Source: CAD feature listing. Evaluate the final solid. Frame: model axes, mm. A direction names the side the tool comes from. Give positions to 0.01 mm unless a question says otherwise; leave off trailing zeros. Order: outer loops, then holes, each group sorted by start corner. A loop starts at its lowest first (then second) coordinate and runs counter-clockwise, first axis right, second up. Notation, with made-up numbers: (16.25, 79) -> (50.25, 79) arc R15 ccw to (50.25, 96) -> close; hole circle Ø6 at (4.25, -32.5). An arc over 180 degrees is marked (long way). Answer in a Markdown table with one row per item.
```python
from build123d import *

# Parameters (mm, degrees)
SKETCH1_W                    = 255
SKETCH1_H                    = 512
BASE_FLANGE1_DEPTH           = 2.3
EDGE_FLANGE2_STRIP_W         = 13.2
EDGE_FLANGE2_STRIP_H         = 2.3
EDGE_FLANGE2_STRIP_CUT_DEPTH = 512
EDGE_FLANGE2_DEPTH           = 512
EDGE_FLANGE3_STRIP_W         = 13.2
EDGE_FLANGE3_STRIP_H         = 2.3
EDGE_FLANGE3_STRIP_CUT_DEPTH = 512
EDGE_FLANGE3_DEPTH           = 512
CUT_EXTRUDE2_START           = -10
CUT_EXTRUDE2_DEPTH           = 586.634510779
EDGE_FLANGE4_STRIP_W         = 13.2
EDGE_FLANGE4_STRIP_H         = 2.3
EDGE_FLANGE4_STRIP_CUT_DEPTH = 246.4
EDGE_FLANGE4_DEPTH           = 246.4
CUT_EXTRUDE3_REACH           = 578.501
SKETCH23_W                   = 219.6
SKETCH23_H                   = 299.3
CUT_EXTRUDE4_REACH           = 578.501
SKETCH24_W                   = 219.6
SKETCH24_H                   = 105
CUT_EXTRUDE6_REACH           = 576.175
SKETCH25_W                   = 55
SKETCH25_H                   = 40
CUT_EXTRUDE7_REACH           = 578.218
SKETCH27_W                   = 16
SKETCH27_H                   = 10
CUT_EXTRUDE8_REACH           = 578.501
SKETCH28_R                   = 5
CUT_EXTRUDE9_REACH           = 578.501
SKETCH29_R                   = 1.75
CUT_EXTRUDE10_REACH          = 578.218
SKETCH30_R                   = 3


# Sheet-metal steps are written as plain solids
with BuildPart() as part:
    # Sketch1 → Base-Flange1 (new body)
    with BuildSketch(Plane.XY):
        with Locations((127.5, 256)):
            Rectangle(SKETCH1_W, SKETCH1_H)
    extrude(amount=-BASE_FLANGE1_DEPTH)

    # Edge-Flange2 strip (across the edge) → Edge-Flange2 strip cut (cut)
    with BuildSketch(Plane(origin=(255, 0, 0), x_dir=(-1, 0, 0), z_dir=(0, 1, 0))):
        with Locations((-2.3, -1.15)):
            Rectangle(EDGE_FLANGE2_STRIP_W, EDGE_FLANGE2_STRIP_H)
    extrude(amount=EDGE_FLANGE2_STRIP_CUT_DEPTH, mode=Mode.SUBTRACT)

    # Edge-Flange2 section (across the edge) → Edge-Flange2 (add)
    with BuildSketch(Plane(origin=(255, 0, 0), x_dir=(-1, 0, 0), z_dir=(0, 1, 0))):
        with BuildLine():
            Line((0, 2), (0, 64.7))
            Line((0, 64.7), (2.3, 64.7))
            Line((2.3, 64.7), (2.3, 2))
            ThreePointArc((2.3, 2), (2.885786438, 0.585786438), (4.3, 0))
            Line((4.3, 0), (4.3, -2.3))
            ThreePointArc((4.3, -2.3), (1.259440841, -1.040559159), (0, 2))
        make_face()
    extrude(amount=EDGE_FLANGE2_DEPTH)

    # Edge-Flange3 strip (across the edge) → Edge-Flange3 strip cut (cut)
    with BuildSketch(Plane.XZ.offset(-512)):
        with Locations((-2.3, -1.15)):
            Rectangle(EDGE_FLANGE3_STRIP_W, EDGE_FLANGE3_STRIP_H)
    extrude(amount=EDGE_FLANGE3_STRIP_CUT_DEPTH, mode=Mode.SUBTRACT)

    # Edge-Flange3 section (across the edge) → Edge-Flange3 (add)
    with BuildSketch(Plane.XZ.offset(-512)):
        with BuildLine():
            Line((0, 2), (0, 64.7))
            Line((0, 64.7), (2.3, 64.7))
            Line((2.3, 64.7), (2.3, 2))
            ThreePointArc((2.3, 2), (2.885786438, 0.585786438), (4.3, 0))
            Line((4.3, 0), (4.3, -2.3))
            ThreePointArc((4.3, -2.3), (1.259440841, -1.040559159), (0, 2))
        make_face()
    extrude(amount=EDGE_FLANGE3_DEPTH)

    # Sketch17 → Cut-Extrude2 (cut)
    with BuildSketch(Plane(origin=(255, 0, 0), x_dir=(0, 0, -1), z_dir=(1, 0, 0)).offset(CUT_EXTRUDE2_START)):
        Polygon((-14.7, -1042.730361711), (-14.7, 0), (-14.7, 300), (-64.7, 512), (-64.7, 0), (-64.7, -1042.730361711), (-64.7, -3128.191085133), (-14.7, -3128.191085133), align=None)
    cut_extrude2 = extrude(amount=CUT_EXTRUDE2_DEPTH, mode=Mode.SUBTRACT)

    # Mirror6: Cut-Extrude2 across plane
    add(cut_extrude2.mirror(Plane(origin=(126.35, 0, 0), x_dir=(0, 0, 1), z_dir=(1, 0, 0))), mode=Mode.SUBTRACT)

    # Edge-Flange4 strip (across the edge) → Edge-Flange4 strip cut (cut)
    with BuildSketch(Plane(origin=(250.7, 512, 0), x_dir=(0, -1, 0), z_dir=(-1, 0, 0))):
        with Locations((-2.3, -1.15)):
            Rectangle(EDGE_FLANGE4_STRIP_W, EDGE_FLANGE4_STRIP_H)
    extrude(amount=EDGE_FLANGE4_STRIP_CUT_DEPTH, mode=Mode.SUBTRACT)

    # Edge-Flange4 section (across the edge) → Edge-Flange4 (add)
    with BuildSketch(Plane(origin=(250.7, 512, 0), x_dir=(0, -1, 0), z_dir=(-1, 0, 0))):
        with BuildLine():
            Line((0, 2), (0, 69.7))
            Line((0, 69.7), (2.3, 69.7))
            Line((2.3, 69.7), (2.3, 2))
            ThreePointArc((2.3, 2), (2.885786438, 0.585786438), (4.3, 0))
            Line((4.3, 0), (4.3, -2.3))
            ThreePointArc((4.3, -2.3), (1.259440841, -1.040559159), (0, 2))
        make_face()
    extrude(amount=EDGE_FLANGE4_DEPTH)

    # Sketch23 → Cut-Extrude3 (cut, up to next)
    with BuildSketch(Plane(origin=(0, 0, -2.3), x_dir=(-1, 0, 0), z_dir=(0, 0, -1)), mode=Mode.PRIVATE) as cut_extrude3_sk1:
        with Locations((-127.5, 209.65)):
            Rectangle(SKETCH23_W, SKETCH23_H)
    cut_extrude3_tool1 = extrude(cut_extrude3_sk1.sketch, amount=-CUT_EXTRUDE3_REACH, mode=Mode.PRIVATE) & part.part
    add(cut_extrude3_tool1.solids().sort_by_distance((127.5, 209.65, -2.3))[0], mode=Mode.SUBTRACT)

    # Sketch24 → Cut-Extrude4 (cut, up to next)
    with BuildSketch(Plane(origin=(0, 0, -2.3), x_dir=(-1, 0, 0), z_dir=(0, 0, -1)), mode=Mode.PRIVATE) as cut_extrude4_sk1:
        with Locations((-127.5, 437.8)):
            Rectangle(SKETCH24_W, SKETCH24_H)
    cut_extrude4_tool1 = extrude(cut_extrude4_sk1.sketch, amount=-CUT_EXTRUDE4_REACH, mode=Mode.PRIVATE) & part.part
    add(cut_extrude4_tool1.solids().sort_by_distance((127.5, 437.8, -2.3))[0], mode=Mode.SUBTRACT)

    # Sketch25 → Cut-Extrude6 (cut, up to next)
    with BuildSketch(Plane.XZ.offset(-509.7), mode=Mode.PRIVATE) as cut_extrude6_sk1:
        with Locations((127.5, 49.7)):
            Rectangle(SKETCH25_W, SKETCH25_H)
    cut_extrude6_tool1 = extrude(cut_extrude6_sk1.sketch, amount=-CUT_EXTRUDE6_REACH, mode=Mode.PRIVATE) & part.part
    add(cut_extrude6_tool1.solids().sort_by_distance((127.5, 509.7, 49.7))[0], mode=Mode.SUBTRACT)

    # Sketch27 → Cut-Extrude7 (cut, up to next)
    with BuildSketch(Plane(origin=(0, 512, 0), x_dir=(1, 0, 0), z_dir=(0, 1, 0)), mode=Mode.PRIVATE) as cut_extrude7_sk1:
        with Locations((108, -2.7)):
            Rectangle(SKETCH27_W, SKETCH27_H)
    cut_extrude7_tool1 = extrude(cut_extrude7_sk1.sketch, amount=-CUT_EXTRUDE7_REACH, mode=Mode.PRIVATE) & part.part
    # Sketch27 → Cut-Extrude7 (cut, up to next)
    with BuildSketch(Plane(origin=(0, 512, 0), x_dir=(1, 0, 0), z_dir=(0, 1, 0)), mode=Mode.PRIVATE) as cut_extrude7_sk2:
        with Locations((147, -2.7)):
            Rectangle(SKETCH27_W, SKETCH27_H)
    cut_extrude7_tool2 = extrude(cut_extrude7_sk2.sketch, amount=-CUT_EXTRUDE7_REACH, mode=Mode.PRIVATE) & part.part
    add(cut_extrude7_tool1.solids().sort_by_distance((108, 512, 2.7))[0], mode=Mode.SUBTRACT)
    add(cut_extrude7_tool2.solids().sort_by_distance((147, 512, 2.7))[0], mode=Mode.SUBTRACT)

    # Sketch28 → Cut-Extrude8 (cut, up to next)
    with BuildSketch(Plane(origin=(0, 0, -2.3), x_dir=(-1, 0, 0), z_dir=(0, 0, -1)), mode=Mode.PRIVATE) as cut_extrude8_sk1:
        with Locations((-127.5, 496)):
            Circle(SKETCH28_R)
    cut_extrude8_tool1 = extrude(cut_extrude8_sk1.sketch, amount=-CUT_EXTRUDE8_REACH, mode=Mode.PRIVATE) & part.part
    add(cut_extrude8_tool1.solids().sort_by_distance((127.5, 496, -2.3))[0], mode=Mode.SUBTRACT)

    # Sketch29 → Cut-Extrude9 (cut, up to next)
    with BuildSketch(Plane(origin=(0, 0, -2.3), x_dir=(-1, 0, 0), z_dir=(0, 0, -1)), mode=Mode.PRIVATE) as cut_extrude9_sk1:
        with Locations((-119.46, 496)):
            Circle(SKETCH29_R)
    cut_extrude9_tool1 = extrude(cut_extrude9_sk1.sketch, amount=-CUT_EXTRUDE9_REACH, mode=Mode.PRIVATE) & part.part
    # Sketch29 → Cut-Extrude9 (cut, up to next)
    with BuildSketch(Plane(origin=(0, 0, -2.3), x_dir=(-1, 0, 0), z_dir=(0, 0, -1)), mode=Mode.PRIVATE) as cut_extrude9_sk2:
        with Locations((-135.54, 496)):
            Circle(SKETCH29_R)
    cut_extrude9_tool2 = extrude(cut_extrude9_sk2.sketch, amount=-CUT_EXTRUDE9_REACH, mode=Mode.PRIVATE) & part.part
    add(cut_extrude9_tool1.solids().sort_by_distance((119.46, 496, -2.3))[0], mode=Mode.SUBTRACT)
    add(cut_extrude9_tool2.solids().sort_by_distance((135.54, 496, -2.3))[0], mode=Mode.SUBTRACT)

    # Sketch30 → Cut-Extrude10 (cut, up to next)
    with BuildSketch(Plane(origin=(0, 512, 0), x_dir=(1, 0, 0), z_dir=(0, 1, 0)), mode=Mode.PRIVATE) as cut_extrude10_sk1:
        with Locations(Location((20.3, -9.700000578, 0), (0, 0, 270))):
            Circle(SKETCH30_R)
    cut_extrude10_tool1 = extrude(cut_extrude10_sk1.sketch, amount=-CUT_EXTRUDE10_REACH, mode=Mode.PRIVATE) & part.part
    # Sketch30 → Cut-Extrude10 (cut, up to next)
    with BuildSketch(Plane(origin=(0, 512, 0), x_dir=(1, 0, 0), z_dir=(0, 1, 0)), mode=Mode.PRIVATE) as cut_extrude10_sk2:
        with Locations(Location((73.3, -9.700000578, 0), (0, 0, 270))):
            Circle(SKETCH30_R)
    cut_extrude10_tool2 = extrude(cut_extrude10_sk2.sketch, amount=-CUT_EXTRUDE10_REACH, mode=Mode.PRIVATE) & part.part
    # Sketch30 → Cut-Extrude10 (cut, up to next)
    with BuildSketch(Plane(origin=(0, 512, 0), x_dir=(1, 0, 0), z_dir=(0, 1, 0)), mode=Mode.PRIVATE) as cut_extrude10_sk3:
        with Locations(Location((20.306798441, -49.7, 0), (0, 0, 270))):
            Circle(SKETCH30_R)
    cut_extrude10_tool3 = extrude(cut_extrude10_sk3.sketch, amount=-CUT_EXTRUDE10_REACH, mode=Mode.PRIVATE) & part.part
    # Sketch30 → Cut-Extrude10 (cut, up to next)
    with BuildSketch(Plane(origin=(0, 512, 0), x_dir=(1, 0, 0), z_dir=(0, 1, 0)), mode=Mode.PRIVATE) as cut_extrude10_sk4:
        with Locations(Location((73.306798441, -49.7, 0), (0, 0, 270))):
            Circle(SKETCH30_R)
    cut_extrude10_tool4 = extrude(cut_extrude10_sk4.sketch, amount=-CUT_EXTRUDE10_REACH, mode=Mode.PRIVATE) & part.part
    # Sketch30 → Cut-Extrude10 (cut, up to next)
    with BuildSketch(Plane(origin=(0, 512, 0), x_dir=(1, 0, 0), z_dir=(0, 1, 0)), mode=Mode.PRIVATE) as cut_extrude10_sk5:
        with Locations(Location((181.693201559, -49.7, 0), (0, 0, 90))):
            Circle(SKETCH30_R)
    cut_extrude10_tool5 = extrude(cut_extrude10_sk5.sketch, amount=-CUT_EXTRUDE10_REACH, mode=Mode.PRIVATE) & part.part
    # Sketch30 → Cut-Extrude10 (cut, up to next)
    with BuildSketch(Plane(origin=(0, 512, 0), x_dir=(1, 0, 0), z_dir=(0, 1, 0)), mode=Mode.PRIVATE) as cut_extrude10_sk6:
        with Locations(Location((234.693201559, -49.7, 0), (0, 0, 90))):
            Circle(SKETCH30_R)
    cut_extrude10_tool6 = extrude(cut_extrude10_sk6.sketch, amount=-CUT_EXTRUDE10_REACH, mode=Mode.PRIVATE) & part.part
    # Sketch30 → Cut-Extrude10 (cut, up to next)
    with BuildSketch(Plane(origin=(0, 512, 0), x_dir=(1, 0, 0), z_dir=(0, 1, 0)), mode=Mode.PRIVATE) as cut_extrude10_sk7:
        with Locations(Location((181.7, -9.700000578, 0), (0, 0, 90))):
            Circle(SKETCH30_R)
    cut_extrude10_tool7 = extrude(cut_extrude10_sk7.sketch, amount=-CUT_EXTRUDE10_REACH, mode=Mode.PRIVATE) & part.part
    # Sketch30 → Cut-Extrude10 (cut, up to next)
    with BuildSketch(Plane(origin=(0, 512, 0), x_dir=(1, 0, 0), z_dir=(0, 1, 0)), mode=Mode.PRIVATE) as cut_extrude10_sk8:
        with Locations(Location((234.7, -9.700000578, 0), (0, 0, 90))):
            Circle(SKETCH30_R)
    cut_extrude10_tool8 = extrude(cut_extrude10_sk8.sketch, amount=-CUT_EXTRUDE10_REACH, mode=Mode.PRIVATE) & part.part
    add(cut_extrude10_tool1.solids().sort_by_distance((20.3, 512, 9.700001))[0], mode=Mode.SUBTRACT)
    add(cut_extrude10_tool2.solids().sort_by_distance((73.3, 512, 9.700001))[0], mode=Mode.SUBTRACT)
    add(cut_extrude10_tool3.solids().sort_by_distance((20.306798, 512, 49.7))[0], mode=Mode.SUBTRACT)
    add(cut_extrude10_tool4.solids().sort_by_distance((73.306798, 512, 49.7))[0], mode=Mode.SUBTRACT)
    add(cut_extrude10_tool5.solids().sort_by_distance((181.693202, 512, 49.7))[0], mode=Mode.SUBTRACT)
    add(cut_extrude10_tool6.solids().sort_by_distance((234.693202, 512, 49.7))[0], mode=Mode.SUBTRACT)
    add(cut_extrude10_tool7.solids().sort_by_distance((181.7, 512, 9.700001))[0], mode=Mode.SUBTRACT)
    add(cut_extrude10_tool8.solids().sort_by_distance((234.7, 512, 9.700001))[0], mode=Mode.SUBTRACT)


solid = part.part
```
(1) Section query C-C (x = 223.5). Return the cut outline in (y, z).
A:
| item | result |
|---|---|
| outline | (0, -2.3) -> (60, -2.3) -> (60, 0) -> (0, 0) -> close; (359.3, -2.3) -> (385.3, -2.3) -> (385.3, 0) -> (359.3, 0) -> close; (490.3, -2.3) -> (507.7, -2.3) arc R4.3 ccw to (512, 2) -> (512, 69.7) -> (509.7, 69.7) -> (509.7, 2) arc R2 cw to (507.7, 0) -> (490.3, 0) -> close |
(2) Ray query, probe 1 along X at (y, z) = (111.5, 6); probe 2 along Y at (x, z) = (135.54, -1.75); probe 3 along Z at (x, y) = (181.7, 510.55). Return the intervals inside material, ascending.
A:
| item | result |
|---|---|
| probe 1 | x = 0 to 2.3, 252.7 to 255 |
| probe 2 | y = 0 to 60, 359.3 to 385.3, 490.3 to 494.25, 497.75 to 509.8 |
| probe 3 | z = -1.22 to 6.7, 12.7 to 46.7, 52.7 to 69.7 |
(3) First-contact query: pin 1 Ø0.7 at (x, y) = (107.5, 511) entering from -Z; pin 2 Ø0.7 at (y, z) = (509.5, -1.5) entering from -X; pin 3 Ø8 at (x, z) = (20.31, 49.7) entering from -Y. Flat tips, straight axial feed; report the tip coordinate or a pass-through.
A:
| item | result |
|---|---|
| pin 1 | stops at z = 7.7 |
| pin 2 | stops at x = 1.37 |
| pin 3 | stops at y = 509.7 |
(4) Section query D-D (y = 309). Return the cut outline in (x, z).
A:
| item | result |
|---|---|
| outline | (0, 2) arc R4.3 ccw to (4.3, -2.3) -> (17.7, -2.3) -> (17.7, 0) -> (4.3, 0) arc R2 cw to (2.3, 2) -> (2.3, 16.82) -> (0, 16.82) -> close; (237.3, -2.3) -> (250.7, -2.3) arc R4.3 ccw to (255, 2) -> (255, 16.82) -> (252.7, 16.82) -> (252.7, 2) arc R2 cw to (250.7, 0) -> (237.3, 0) -> close |
(5) Section query A-A (x = 127.5). Return the cut outline in (y, z), plus the area to 3 significant figures.
A:
| item | result |
|---|---|
| outline | (0, -2.3) -> (60, -2.3) -> (60, 0) -> (0, 0) -> close; (359.3, -2.3) -> (385.3, -2.3) -> (385.3, 0) -> (359.3, 0) -> close; (490.3, -2.3) -> (491, -2.3) -> (491, 0) -> (490.3, 0) -> close; (501, -2.3) -> (507.7, -2.3) arc R4.3 ccw to (512, 2) -> (512, 29.7) -> (509.7, 29.7) -> (509.7, 2) arc R2 cw to (507.7, 0) -> (501, 0) -> close |
| area | 290 mm^2 |
(6) Access query for faces 4 (the flat face through (252.7, 309, 13)), 5 (the flat face through (17, 199, 0)), 6 (the flat face through (100, 503.6, -0.2)), 7 (the flat face through (129, 512, 28)). Directions: +Z, -Z, +X, -X, +Y, -Y. A direction counts if a zero-diameter tool reaches every point of the face in a straight line with its end or side. Return the directions, or none.
A:
| item | result |
|---|---|
| face 4 | +Z, +Y, -Y |
| face 5 | +Z, -Y |
| face 6 | -Z, +Y |
| face 7 | +Z, -Z, +X, -X, +Y |
(7) Pull-direction query (Y, two-part tool) for faces 1 (the cylindrical face through (124.812, 500.216, -1.166)), 2 (the flat face through (130, 501, 0)), 3 (the flat face through (253.83, 404.52, 39.35)); classes: +Y half, -Y half, draft (parallel to the pull), parting line (faces both ways), or undercut.
A:
| item | result |
|---|---|
| face 1 | undercut |
| face 2 | draft |
| face 3 | -Y half |
(8) Section query B-B (y = 402). Return the cut outline in (x, z).
A:
| item | result |
|---|---|
| outline | (0, 2) arc R4.3 ccw to (4.3, -2.3) -> (17.7, -2.3) -> (17.7, 0) -> (4.3, 0) arc R2 cw to (2.3, 2) -> (2.3, 38.76) -> (0, 38.76) -> close; (237.3, -2.3) -> (250.7, -2.3) arc R4.3 ccw to (255, 2) -> (255, 38.76) -> (252.7, 38.76) -> (252.7, 2) arc R2 cw to (250.7, 0) -> (237.3, 0) -> close |
